from build123d import *

# Parameters (mm, degrees)
SKETCH1_R           = 5.334
SKETCH1_R_2         = 4.064
BOSS_EXTRUDE1_DEPTH = 120.396
BOSS_EXTRUDE2_START = 0.508
SKETCH2_R           = 8.6995
SKETCH2_R_2         = 4.064
BOSS_EXTRUDE2_DEPTH = 0.508


with BuildPart() as part:
    # Sketch1 → Boss-Extrude1 (new body)
    with BuildSketch(Plane(origin=(0, 0, 0), x_dir=(1, 0, 0), z_dir=(0, 1, 0))):
        with Locations(Location((0, 0, 0), (0, 0, 90))):
            Circle(SKETCH1_R)
        with Locations(Location((0, 0, 0), (0, 0, 90))):
            Circle(SKETCH1_R_2, mode=Mode.SUBTRACT)
    extrude(amount=BOSS_EXTRUDE1_DEPTH)

    # Sketch2 → Boss-Extrude2 (add)
    with BuildSketch(Plane.XZ.offset(BOSS_EXTRUDE2_START)):
        with Locations(Location((0, 0, 0), (0, 0, 270))):
            Circle(SKETCH2_R)
        with Locations(Location((0, 0, 0), (0, 0, 270))):
            Circle(SKETCH2_R_2, mode=Mode.SUBTRACT)
    extrude(amount=-BOSS_EXTRUDE2_DEPTH)


solid = part.part
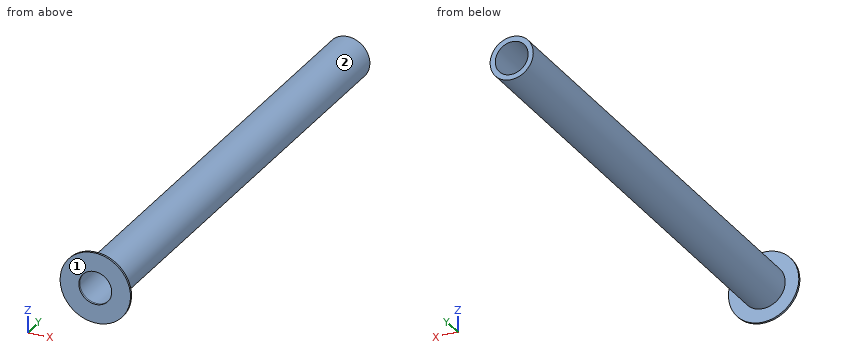
The model under review builds one solid part; all positions refer to its coordinate system, in mm. Face numbers are marked on the shaded views. A direction names the side the tool comes from. Round coordinates to 2 decimals unless told otherwise and drop trailing zeros. Loops run counter-clockwise (first coordinate to the right, second up) from the corner with the lowest first, then second, coordinate; pieces in that order, holes last. Notation, with made-up numbers: (30, 7) -> (56, 7) arc R19 ccw to (56, 32) -> close; hole circle Ø1 at (11, 43.5). An arc over 180 degrees is marked (long way). Return JSON: item names as keys, results as strings.
(1) Add section D-D on z = 7.25. Write out the cut boundary in (x, y), plus the area to 3 significant figures.
Solved:
{"outline": "(-4.81, -0.51) -> (4.81, -0.51) -> (4.81, 0) -> (-4.81, 0) -> close", "area": "4.89 mm2"}
(2) Add section C-C on y = 96. Write out the cut boundary in (x, z).
Solved:
{"outline": "circle Ø10.67 at (0, 0); hole circle Ø8.13 at (0, 0)"}
(3) For the marked faces 1 and 2, list the 3-axis set-ups (+Z, -Z, +X, -X, +Y, -Y) from which the entire face can be reached by the end or side of a thin tool; tool diameter is ignored.
Solved:
{"face 1": "+Z, -Z, +X, -X, -Y", "face 2": "+Y"}
(4) For line 1 (X direction, y = 91, z = 0); line 2 (X direction, y = -0.4, z = 0); line 3 (Y direction, x = 6.5, z = -2.5), list the stretches that pass through material, from the lowest coordinate up.
Solved:
{"line 1": "-5.33 to -4.06, 4.06 to 5.33", "line 2": "-8.7 to -4.06, 4.06 to 8.7", "line 3": "-0.51 to 0"}
(5) For pin 1 (8 mm diameter, centred on x = 2.5, y = 102.5, fed in from +Z); pin 2 (3 mm diameter, centred on x = 0, y = 39.5, fed in from -Z); pin 3 (6 mm diameter, centred on y = 34.5, z = 4.5, fed in from -X), all flat-tipped, find the tip position at first contact; note any pin that passes through.
Solved:
{"pin 1": "z = 5.33", "pin 2": "z = -5.33", "pin 3": "x = -5.12"}
(6) Add section B-B on z = 0. Write out the cut boundary in (x, y), plus the area to 3 significant figures.
Solved:
{"outline": "(-8.7, -0.51) -> (-4.06, -0.51) -> (-4.06, 120.4) -> (-5.33, 120.4) -> (-5.33, 0) -> (-8.7, 0) -> close; (4.06, -0.51) -> (8.7, -0.51) -> (8.7, 0) -> (5.33, 0) -> (5.33, 120.4) -> (4.06, 120.4) -> close", "area": "311 mm2"}
(7) Add section A-A on x = 0. Write out the cut boundary in (y, z), plus the area to 3 significant figures.
Solved:
{"outline": "(-0.51, -8.7) -> (0, -8.7) -> (0, -5.33) -> (120.4, -5.33) -> (120.4, -4.06) -> (-0.51, -4.06) -> close; (-0.51, 4.06) -> (120.4, 4.06) -> (120.4, 5.33) -> (0, 5.33) -> (0, 8.7) -> (-0.51, 8.7) -> close", "area": "311 mm2"}
